Could you check a few things on this drawing? It's one solid part, dimensions in mm from its lowest x, y, z. A direction names the side the tool comes from. Give positions to 0.01 mm unless a question says otherwise; leave off trailing zeros. Order: outer loops, then holes, each group sorted by start corner. A loop starts at its lowest first (then second) coordinate and runs counter-clockwise, first axis right, second up. Notation, with made-up numbers: (-7, 17.5) - (12, 17.5) arc R16 cw to (12, 40.5) - close; hole circle Ø11 at (40, -21.5). An arc over 180 degrees is marked (long way). Put each result on its own line as item: value.
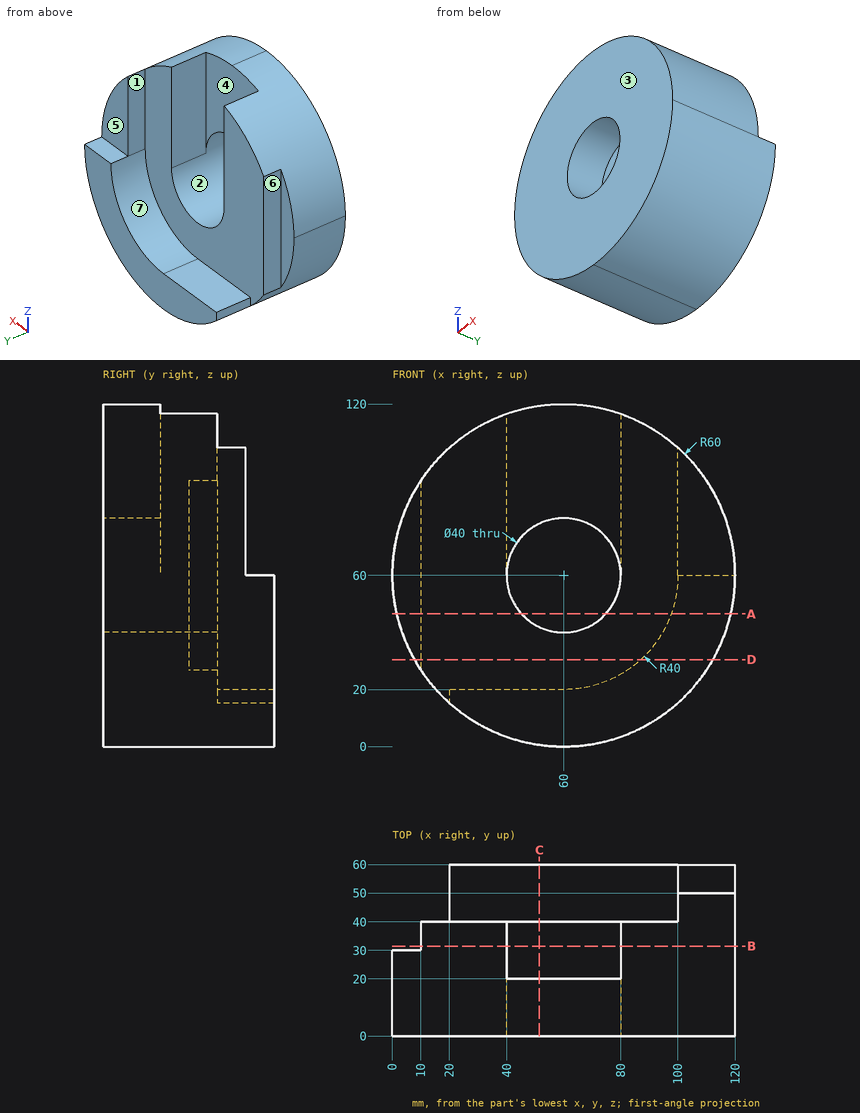
1) We'd pull the mould along X, two halves only. Please class the marked faces 1, 2 and 3: pulls with the +X half, pulls with the -X half, needs draft (parallel to the pull), parting line crosses it, or undercut.
Filled in:
face 1: pulls with the -X half
face 2: undercut
face 3: needs draft
2) Suppose I cut it at C-C, the plane x = 51.5. List the corners of the cut face in (y, z) for me.
Filled in:
outline: (0, 0.61) - (60, 0.61) - (60, 20) - (40, 20) - (40, 41.9) - (0, 41.9) - close; (0, 78.1) - (20, 78.1) - (20, 119.39) - (0, 119.39) - close
3) I'm going to push flat-ended pins straight in: pin 1 (8 mm diameter, centred on y = 14, z = 19, fed in from +X); pin 2 (4 mm diameter, centred on y = 47, z = 17.5, fed in from -X); pin 3 (20 mm diameter, centred on x = 61.5, z = 90.5, fed in from +Y); pin 4 (1 mm diameter, centred on x = 91, z = 42, fed in from -Y). Where does each tip first touch, or does it pass through?
Filled in:
pin 1: stops at x = 107.23
pin 2: stops at x = 20
pin 3: stops at y = 20
pin 4: stops at y = 0
4) Which directions (+Z, -Z, +X, -X, +Y, -Y) give clear straight access to the entire face, cutting with the end or side of a thin tool? Please do the marked faces 4, 5, 6 and 7.
Filled in:
face 4: +Z, +Y
face 5: +Z, +X, -X, +Y
face 6: +Z, -Z, -X, +Y
face 7: +Z, -X, +Y
5) Suppose I cut it at A-A, the plane z = 46.5. List the corners of the cut face in (x, y) for me.
Filled in:
outline: (1.54, 0) - (45.24, 0) - (45.24, 40) - (10, 40) - (10, 30) - (1.54, 30) - close; (74.76, 0) - (118.46, 0) - (118.46, 60) - (97.65, 60) - (97.65, 40) - (74.76, 40) - close
6) Suppose I cut it at B-B, the plane y = 31.5. List the corners of the cut face in (x, z) for me.
Filled in:
outline: (10, 26.83) arc R60 ccw (long way) to (80, 116.57) - (80, 60) arc R20 cw to (40, 60) - (40, 116.57) arc R60 ccw to (10, 93.17) - close
7) Suppose I cut it at D-D, the plane z = 30.5. List the corners of the cut face in (x, y) for me, and give its area (3 significant figures).
Filled in:
outline: (7.75, 0) - (112.25, 0) - (112.25, 60) - (87.01, 60) - (87.01, 40) - (10, 40) - (10, 30) - (7.75, 30) - close
area: 4,660 mm^2
8) If I drill on line 1 (Z direction, x = 60, y = 9); line 2 (Y direction, x = 36.5, z = 95.5), over which ranges is the centre line in solid material (lowest first)? Write a range as [from, to].
Filled in:
line 1: z = [0, 40], [80, 120]
line 2: y = [0, 40]
